```python
from build123d import *

# Parameters (mm, degrees)
F0_R     = 2
F1_DEPTH = 0.8


with BuildPart() as f1:
    # F0 (on Top) → F1 (new body)
    with BuildSketch(Plane.XY):
        with BuildLine():
            Line((0, -6.35), (101.6, -6.35))
            ThreePointArc((101.6, -6.35), (106.090128, -4.490128), (107.95, 0))
            ThreePointArc((107.95, 0), (106.090128, 4.490128), (101.6, 6.35))
            Line((101.6, 6.35), (0, 6.35))
            ThreePointArc((0, 6.35), (-4.490128, 4.490128), (-6.35, 0))
            ThreePointArc((-6.35, 0), (-4.490128, -4.490128), (0, -6.35))
        make_face()
        Circle(F0_R, mode=Mode.SUBTRACT)
        with Locations((12.7, 0)):
            Circle(F0_R, mode=Mode.SUBTRACT)
        with Locations((25.4, 0)):
            Circle(F0_R, mode=Mode.SUBTRACT)
        with Locations((38.1, 0)):
            Circle(F0_R, mode=Mode.SUBTRACT)
        with Locations((50.8, 0)):
            Circle(F0_R, mode=Mode.SUBTRACT)
        with Locations((63.5, 0)):
            Circle(F0_R, mode=Mode.SUBTRACT)
        with Locations((76.2, 0)):
            Circle(F0_R, mode=Mode.SUBTRACT)
        with Locations((88.9, 0)):
            Circle(F0_R, mode=Mode.SUBTRACT)
        with Locations((101.6, 0)):
            Circle(F0_R, mode=Mode.SUBTRACT)
    extrude(amount=F1_DEPTH)


solid = f1.part
```
The listing builds one solid part. Answer for the finished solid, in the listing's coordinates (mm). Coordinates: 2 decimals unless noted, no trailing zeros. Loops run counter-clockwise (first coordinate to the right, second up) from the corner with the lowest first, then second, coordinate; pieces in that order, holes last. Notation, with made-up numbers: M 82.25,18 L 125.25,18 A14 cw 125.25,24 Z; hole C -22.5,77.5 d6. An arc over 180 degrees is marked long. Answer as CSV lines item,"result". Start each with the question number.
(1) The part is cut by section D-D (y = 4). Give the vertices of the cut face in (x, z).
(2) The part is cut by section B-B (z = 0.5). State how many separate pieces and enclosed holes the cut face has, and give its area (3 significant figures).
(3) The part is cut by section A-A (x = 63.5). Give the vertices of the cut face in (y, z), and give its area (3 significant figures).
(4) Find the intervals of material crossed by L1, parallel to Y at x = 101.6, z = 0.35; L2, parallel to X at y = -5.25, z = 0.7; L3, parallel to X at y = 3.25, z = 0.1, in increasing order. Write a range as [from, to].
(5) Given pin 1 (2.5 mm diameter, centred on x = 25.4, y = 0, fed in from +Z), flat-ended and moving along its own axis, determine where the tip first touches the part or whether it passes through.
(6) The mould has two halves that part along X. Classify faces 1 (the cylindrical face through (74.202, 0.088, 0.394)), 2 (the flat face through (50, 3, 0)): pulls with the +X half, pulls with the -X half, needs draft (parallel to the pull), parting line crosses it, or undercut.
(7) The part is cut by section C-C (x = 39). Give the vertices of the cut face in (y, z).
Determined:
1,outline,"M -4.93,0 L 106.53,0 L 106.53,0.8 L -4.93,0.8 Z"
2,separate pieces,"1"
2,enclosed holes,"9"
2,area,"1,300 mm2"
3,outline,"M -6.35,0 L -2,0 L -2,0.8 L -6.35,0.8 Z; M 2,0 L 6.35,0 L 6.35,0.8 L 2,0.8 Z"
3,area,"6.96 mm2"
4,L1,"[-6.35, -2], [2, 6.35]"
4,L2,"[-3.57, 105.17]"
4,L3,"[-5.46, 107.06]"
5,pin 1,"through"
6,face 1,"undercut"
6,face 2,"needs draft"
7,outline,"M -6.35,0 L -1.79,0 L -1.79,0.8 L -6.35,0.8 Z; M 1.79,0 L 6.35,0 L 6.35,0.8 L 1.79,0.8 Z"
